Autodesk Inventor part; units mm, degrees
ref_plane "YZ Plane" through (0, 0, 0) normal (1, 0, 0) x (0, 1, 0)
ref_plane "XZ Plane" through (0, 0, 0) normal (0, 1, 0) x (-1, 0, 0)
ref_plane "XY Plane" through (0, 0, 0) normal (0, 0, 1) x (1, 0, 0)
sketch "Sketch1" plane through (0, 0, 0) normal (1, 0, 0) x (0, 1, 0)
  circle A0 centre (0, 0) radius 2.1844
  circle A1 centre (0, 0) radius 3.81
  circle A2 centre (3.8397, 28.1547) radius 2.1844
  circle A3 centre (3.8397, 28.1547) radius 5.08
  line L0 (0, 0) -> (16.51, 0) construction
  circle A4 centre (17.5016, -4.6538) radius 2.1844
  line L1 (0, 0) -> (16.51, 0) construction
  circle A5 centre (4.5215, 17.5685) radius 2.1844
  circle A6 centre (4.5215, 17.5685) radius 3.81
  circle A7 centre (17.5016, -4.6538) radius 3.81
  line L2 (0, 0) -> (12.7, 0) construction
  line L3 (-0.9791, -3.6821) -> (16.5226, -8.3359)
  line L4 (8.5961, 29.9387) -> (21.069, -3.3158)
  arc A8 (-3.5374, 1.4152) -> (-1.1438, 27.1693) centre (-45.8278, 18.334) ccw
  point P0 (-1.2195, 28.6143)
  point P1 (-3.7944, 0.3447)
  dimension "d0" = 4.3688
  dimension "d1" = 7.62
  dimension "d3" = 4.3688
  dimension "d4" = 10.16
  dimension "d8" = 4.3688
  dimension "d11" = 4.3688
  dimension "d12" = 7.62
  dimension "d13" = 7.62
extrude "Extrusion1" add sketch "Sketch1" along normal blind 1.5875 contours A1 | A1 A8 A3 L4 A7 L3 | A3 | A7 | A6
properties part number "rotationmount"
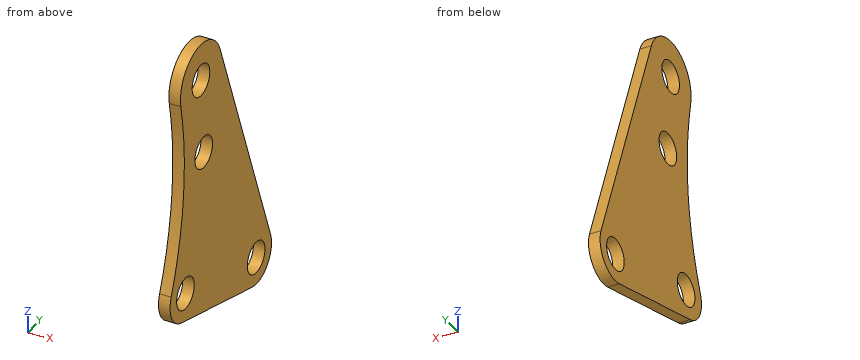
Verification items for the finished model (mm, model axes). Give positions to 0.01 mm unless a question says otherwise; leave off trailing zeros. Write each loop counter-clockwise with the first axis right and the second up, starting at its lowest first coordinate (ties: lowest second). Pieces come first, ordered by that corner, then holes. Notation, with made-up numbers: (20.25, -40) - (44.25, -40) arc R8 ccw to (44.25, -34) - close; hole circle Ø8 at (87, 50.5). An arc over 180 degrees is marked (long way). Put each result on its own line as item: value.
Q1. Section check B-B on z = 0. Record the cut outline in (x, y).
Result:
outline: (0, -3.81) - (1.59, -3.81) - (1.59, -2.18) - (0, -2.18) - close; (0, 2.18) - (1.59, 2.18) - (1.59, 19.83) - (0, 19.83) - close
Q2. Section check D-D on z = 23. Record the cut outline in (x, y).
Result:
outline: (0, -0.52) - (1.59, -0.52) - (1.59, 11.2) - (0, 11.2) - close
Q3. Scan lines: probe 1 along Z at (x, y) = (1.3, 5); probe 2 along Z at (x, y) = (0.9, 5.75); probe 3 along Y at (x, z) = (0.75, 29.5). Record each from-to range of solid material in increasing order. Write a range as from..to.
Result:
probe 1: -5.27..15.44, 19.7..26.3, 30.01..33.1
probe 2: -5.47..15.76, 19.37..27.1, 29.21..32.86
probe 3: -1.06..2.12, 5.56..8.76
Q4. Section check A-A on x = 0.3. Record the cut outline in (y, z).
Result:
outline: (-3.54, 1.42) arc R3.81 ccw to (-0.98, -3.68) - (16.52, -8.34) arc R3.81 ccw to (21.07, -3.32) - (8.6, 29.94) arc R5.08 ccw to (-1.14, 27.17) arc R45.55 cw to start; hole circle Ø4.37 at (0, 0); hole circle Ø4.37 at (3.84, 28.15); hole circle Ø4.37 at (4.52, 17.57); hole circle Ø4.37 at (17.5, -4.65)
Q5. Depth check by flat-ended pin: P1, Ø5.5, axis at y = 4.52, z = 17.57, coming from the -X side; P2, Ø3.5, axis at y = 0, z = 0, coming from the -X side. Enter the tip coordinate at first touch or a pass-through.
Result:
P1: x = 0
P2: through
Q6. Section check C-C on z = 16. Record the cut outline in (x, y), and give its area (3 significant figures).
Result:
outline: (0, -0.34) - (1.59, -0.34) - (1.59, 3) - (0, 3) - close; (0, 6.04) - (1.59, 6.04) - (1.59, 13.82) - (0, 13.82) - close
area: 17.7 mm2
